```python
from build123d import *

# Parameters (mm, degrees)
BASE_FLANGE1_DEPTH          = 40
F_3_0MM_PRESS_DOWEL_HOLE1_D = 3
F_3_0MM_PRESS_DOWEL_HOLE2_D = 3


# Sheet-metal steps are written as plain solids
with BuildPart() as part:
    # Sketch1 → Base-Flange1 (new body)
    with BuildSketch(Plane(origin=(0, 0, 0), x_dir=(1, 0, 0), z_dir=(0, 1, 0))):
        with BuildLine():
            Line((0, 0), (22.7634, 0))
            ThreePointArc((22.7634, 0), (24.344915027, -0.655084973), (25, -2.2366))
            Line((25, -2.2366), (25, -39.2634))
            ThreePointArc((25, -39.2634), (25.215745145, -39.784254855), (25.7366, -40))
            Line((25.7366, -40), (40, -40))
            Line((40, -40), (40, -41.5))
            Line((40, -41.5), (25.7366, -41.5))
            ThreePointArc((25.7366, -41.5), (24.155084973, -40.844915027), (23.5, -39.2634))
            Line((23.5, -39.2634), (23.5, -2.2366))
            ThreePointArc((23.5, -2.2366), (23.284254855, -1.715745145), (22.7634, -1.5))
            Line((22.7634, -1.5), (0, -1.5))
            Line((0, -1.5), (0, 0))
        make_face()
    extrude(amount=BASE_FLANGE1_DEPTH)

    # Ø3.0mm Press Dowel Hole1 (through all)
    with Locations(Plane(origin=(0, 0, 40), x_dir=(-1, 0, 0), z_dir=(0, 0, -1))):
        with Locations((-33.705752928, 33.5), (-33.705752928, 6.5)):
            Hole(F_3_0MM_PRESS_DOWEL_HOLE1_D / 2)

    # Ø3.0mm Press Dowel Hole2 (through all)
    with Locations(Plane(origin=(0, 0, 0), x_dir=(-1, 0, 0), z_dir=(0, 0, -1))):
        with Locations((-5.626733286, 35), (-5.626733286, 5), (-5.626733286, 20)):
            Hole(F_3_0MM_PRESS_DOWEL_HOLE2_D / 2)


solid = part.part
```
CAD build for the part. Positions are in the model's coordinates, mm. A direction names the side the tool comes from. Give positions to 0.01 mm unless a question says otherwise; leave off trailing zeros. Write each loop counter-clockwise with the first axis right and the second up, starting at its lowest first coordinate (ties: lowest second). Pieces come first, ordered by that corner, then holes. Notation, with made-up numbers: (-40, 76.25) -> (-5, 76.25) arc R21 cw to (-5, 88.25) -> close; hole circle Ø11 at (70.25, 45.25). An arc over 180 degrees is marked (long way). Write each question's results on one line, items separated by ' | '.
1. Drop flat-ended pins along their axis: P1, Ø8, axis at x = 34, y = 33.5, coming from the -Z side; P2, Ø7, axis at x = 15, y = 24.5, coming from the +Z side; P3, Ø1.5, axis at x = 25.5, y = 24, coming from the -Z side; P4, Ø15.5, axis at x = 30.5, y = 16.5, coming from the -Z side. Give the stop position or say it passes through.
Geometry check:
P1: z = 40 | P2: z = 1.5 | P3: z = 1.21 | P4: z = 0
2. Cut at B-B, the plane x = 34.5. Write the cut outline in (y, z), then the cut area to 3 significant figures.
Geometry check:
outline: (0, 40) -> (5.23, 40) -> (5.23, 41.5) -> (0, 41.5) -> close; (7.77, 40) -> (32.23, 40) -> (32.23, 41.5) -> (7.77, 41.5) -> close; (34.77, 40) -> (40, 40) -> (40, 41.5) -> (34.77, 41.5) -> close | area: 52.4 mm²
3. Which spindle directions (+Z, -Z, +X, -X, +Y, -Y) get a long thin tool onto all of the face, cutting with end or side? Do faces 5 (the flat face through (33, 20, 40)), 6 (the cylindrical face through (5.431, 21.487, 0.76)), 7 (the flat face through (23.5, 20, 21)). Say none if no direction does.
Geometry check:
face 5: -Z, +X, +Y, -Y | face 6: +Z, -Z | face 7: +Z, -X, +Y, -Y
4. Cut at D-D, the plane z = 29.5. Write the cut outline in (x, y), then the cut area to 3 significant figures.
Geometry check:
outline: (23.5, 0) -> (25, 0) -> (25, 40) -> (23.5, 40) -> close | area: 60.0 mm²
5. Wall check: probe 1 along X at (y, z) = (10, 3); probe 2 along Z at (x, y) = (37.5, 8); probe 3 along Z at (x, y) = (15.5, 34.5). Give the ranges that are in metal, low to high. Write a range as [from, to].
Geometry check:
probe 1: [23.5, 25] | probe 2: [40, 41.5] | probe 3: [0, 1.5]
6. Cut at A-A, the plane y = 20. Write the cut outline in (x, z), then the cut area to 3 significant figures.
Geometry check:
outline: (0, 0) -> (4.13, 0) -> (4.13, 1.5) -> (0, 1.5) -> close; (7.13, 0) -> (22.76, 0) arc R2.24 ccw to (25, 2.24) -> (25, 39.26) arc R0.74 cw to (25.74, 40) -> (40, 40) -> (40, 41.5) -> (25.74, 41.5) arc R2.24 ccw to (23.5, 39.26) -> (23.5, 2.24) arc R0.74 cw to (22.76, 1.5) -> (7.13, 1.5) -> close | area: 114 mm²
7. Two-plate mould, pull along X, no slides. Class faces 1 (the cylindrical face through (32.515, 5.587, 40.76)), 2 (the flat face through (40, 20, 41)), 3 (the flat face through (11, 20, 0)), 4 (the cylindrical face through (24.17, 19.72, 40.86)): pulls with the +X half, pulls with the -X half, needs draft (parallel to the pull), parting line crosses it, or undercut.
Geometry check:
face 1: undercut | face 2: pulls with the +X half | face 3: needs draft | face 4: pulls with the -X half
8. Cut at C-C, the plane y = 31. Write the cut outline in (x, z).
Geometry check:
outline: (0, 0) -> (22.76, 0) arc R2.24 ccw to (25, 2.24) -> (25, 39.26) arc R0.74 cw to (25.74, 40) -> (40, 40) -> (40, 41.5) -> (25.74, 41.5) arc R2.24 ccw to (23.5, 39.26) -> (23.5, 2.24) arc R0.74 cw to (22.76, 1.5) -> (0, 1.5) -> close
